Autodesk Inventor part; units mm, degrees
ref_plane "Work Plane1" through (19.05, -6.35, 0) normal (1, 0, 0) x (0, 0, -1)
ref_plane "YZ Plane" through (0, 0, 0) normal (1, 0, 0) x (0, 1, 0)
ref_plane "XZ Plane" through (0, 0, 0) normal (0, 1, 0) x (-1, 0, 0)
sketch "Sketch1" plane through (0, 0, 0) normal (0, 0, 1) x (1, 0, 0)
  line L0 (-6.35, 6.35) -> (6.35, 6.35)
  line L1 (6.35, 6.35) -> (6.35, -6.35)
  line L2 (6.35, -6.35) -> (-6.35, -6.35)
  line L3 (-6.35, -6.35) -> (-6.35, 6.35)
  point P0 (0, 0)
  point P1 (0, 6.35)
  point P2 (-6.35, 0)
  dimension "d0" = 12.7
  dimension "d1" = 12.7
extrude "Extrusion1" add sketch "Sketch1" along normal blind 38.1
ref_plane "Work Plane1" through (19.05, -6.35, 0) normal (1, 0, 0) x (0, 0, -1)
sketch "Sketch2" plane through (19.05, -6.35, 0) normal (1, 0, 0) x (0, 0, -1)
  line L0 (-38.1, 12.7) -> (-38.1, 0)
  line L1 (0, 0) -> (-38.1, 0)
  line L2 (0, 12.7) -> (0, 0)
  line L3 (0, 12.7) -> (-38.1, 12.7)
  line L4 (-38.1, 7.9375) -> (-12.7, 7.9375)
  arc A0 (-12.7, 7.9375) -> (-7.9375, 12.7) centre (-12.7, 12.7) ccw
  point P0 (0, 6.35)
  dimension "d5" = 25.4
  dimension "d6" = 1.5875
  dimension "d7" = 4.7625
extrude "Extrusion2" cut sketch "Sketch2" against normal blind 38.1 contours L3 A0 L4 L0
mirror "Mirror1" about plane through (0, 0, 0) normal (0, 1, 0) of "Extrusion2"
sketch "Sketch3" plane through (19.05, -6.35, 0) normal (1, 0, 0) x (0, 0, -1)
  arc A0 (-7.9375, 0) -> (-12.7, 4.7625) centre (-12.7, 0) ccw
  line L0 (0, 0) -> (-7.9375, 0)
  line L1 (0, 12.7) -> (0, 0)
  line L2 (0, 12.7) -> (-7.9375, 12.7)
  arc A1 (-12.7, 7.9375) -> (-7.9375, 12.7) centre (-12.7, 12.7) ccw
  line L3 (-12.7, 7.9375) -> (-38.1, 7.9375)
  line L4 (-38.1, 7.9375) -> (-38.1, 4.7625)
  line L5 (-38.1, 4.7625) -> (-12.7, 4.7625)
  line L6 (-30.48, 7.9375) -> (-30.48, 6.35)
  line L7 (-30.48, 6.35) -> (-38.1, 6.35)
  point P0 (0, 6.35)
  dimension "d10" = 1.5875
  dimension "d11" = 7.62
extrude "Extrusion3" cut sketch "Sketch3" against normal blind 38.1 contours L4 L3 L6 L7
sketch "Sketch4" plane through (-6.35, 0, 30.48) normal (0, 1, 0) x (1, 0, 0)
  line L0 (0, -7.62) -> (0, 0)
  line L1 (12.7, -7.62) -> (0, -7.62)
  point P0 (6.35, 30.48)
  point P1 (6.35, -5.08)
  dimension "d14" = 6.35
  dimension "d15" = 2.54
hole "Hole1" at (0, 0, 35.56) direction (0, -1, 0) diameter 2.159 end through all
sketch "Sketch5" plane through (0, 0, 0) normal (0, 0, -1) x (-1, 0, 0)
  point P0 (0, 0)
  point P1 (0, 0)
hole "Hole2" at (0, 0, 0) direction (0, 0, 1) diameter 3.302 depth 7.62 tip angle 118
properties part number "headplateHolder"
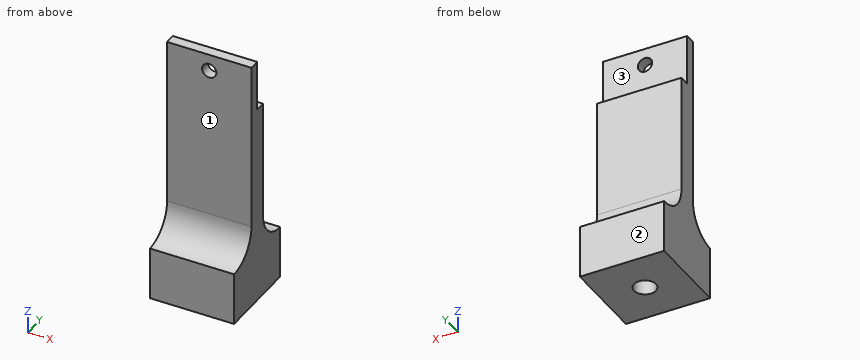
Can you work these out from the model? Positions are in its coordinate system, mm. Face numbers are marked on the shaded views. A direction names the side the tool comes from. Give positions to 0.01 mm unless a question says otherwise; leave off trailing zeros. Loops run counter-clockwise (first coordinate to the right, second up) from the corner with the lowest first, then second, coordinate; pieces in that order, holes last. Notation, with made-up numbers: M -37.75,15 L -16.75,15 A31 cw -16.75,44 Z; hole C 25,2.5 d2. An arc over 180 degrees is marked long. One line per item, written item: value.
1) Imagine slicing it at D-D on y = -5.25. Write out the boundary of the cut face in (x, z), and give its area (3 significant figures).
Geometry check:
outline: M -6.35,0 L 6.35,0 L 6.35,8.07 L -6.35,8.07 Z
area: 102 mm²
2) On a 3-axis mill with a long thin cutter (end or side, diameter ignored), from which of +Z, -Z, +X, -X, +Y, -Y can I reach the whole of each face in a straight line? I mean the marked faces 1, 2 and 3. Say none if no direction works.
Geometry check:
face 1: +Z, +X, -X, -Y
face 2: +Z, -Z, +X, -X, +Y
face 3: +Z, +X, -X, +Y
3) I'm going to push flat-ended pins straight in: pin 1 (4 mm diameter, centred on x = 0, z = 29, fed in from -Y); pin 2 (3 mm diameter, centred on x = -3.5, z = 23, fed in from +Y); pin 3 (1 mm diameter, centred on x = -1.5, z = 9, fed in from +Y). Where does each tip first touch, or does it pass through?
Geometry check:
pin 1: stops at y = -1.59
pin 2: stops at y = 1.59
pin 3: stops at y = 4.1
4) Imagine slicing it at A-A on z = 7. Write out the boundary of the cut face in (x, y).
Geometry check:
outline: M -6.35,-6.35 L 6.35,-6.35 L 6.35,6.35 L -6.35,6.35 Z; hole C 0,0 d3.3
5) Please list where these lines run through material, in increasing order: line 1 (X direction, y = 0, z = 6); line 2 (X direction, y = -0.9, z = 35.56).
Geometry check:
line 1: x = -6.35 to -1.65, 1.65 to 6.35
line 2: x = -6.35 to -1.08, 1.08 to 6.35
6) Imagine slicing it at B-B on z = 35.56. Write out the boundary of the cut face in (x, y), and give its area (3 significant figures).
Geometry check:
outline: M -6.35,-1.59 L -1.08,-1.59 L -1.08,0 L -6.35,0 Z; M 1.08,-1.59 L 6.35,-1.59 L 6.35,0 L 1.08,0 Z
area: 16.7 mm²
